```python
from build123d import *

# Parameters (mm, degrees)
CHAMFER1_SIZE       = 1
CHAMFER2_SIZE       = 0.5
SKETCH2_OUTSIDE_W   = 43.394
SKETCH2_OUTSIDE_H   = 43.394
SKETCH2_OUTSIDE_W_2 = 33.661520222
SKETCH2_OUTSIDE_H_2 = 15
CUT_EXTRUDE1_DEPTH  = 6


with BuildPart() as part:
    # Sketch1 → Revolve1 (revolve)
    with BuildSketch(Plane.XY):
        Polygon((3.5, -5), (3.5, 56), (6.5, 56), (6.5, 46), (10, 46), (10, 4), (13.5, 4), (13.5, 0), (6.25, 0), (6.25, -5), align=None)
    revolve(axis=Axis((0, 0, 0), (0, 1, 0)))

    # Chamfer1
    chamfer1_edges = [part.edges().sort_by_distance(p)[0] for p in [
        (-6.5, 56, 0),
    ]]
    chamfer(chamfer1_edges, length=CHAMFER1_SIZE)

    # Chamfer2
    chamfer2_edges = [part.edges().sort_by_distance(p)[0] for p in [
        (-10, 46, 0),
        (-3.5, 56, 0),
        (-3.5, -5, 0),
        (-6.25, -5, 0),
        (-13.5, 0, 0),
        (-13.5, 4, 0),
    ]]
    chamfer(chamfer2_edges, length=CHAMFER2_SIZE)

    # Sketch2 outside → Cut-Extrude1 (cut)
    with BuildSketch(Plane(origin=(0, 4, 0), x_dir=(1, 0, 0), z_dir=(0, 1, 0))):
        Rectangle(SKETCH2_OUTSIDE_W, SKETCH2_OUTSIDE_H)
        Rectangle(SKETCH2_OUTSIDE_W_2, SKETCH2_OUTSIDE_H_2, mode=Mode.SUBTRACT)
    extrude(amount=CUT_EXTRUDE1_DEPTH, mode=Mode.SUBTRACT)


solid = part.part
```
Check sheet for the modelled part. Datum: model origin and axes. Units: mm. A direction names the side the tool comes from. Give positions to 0.01 mm unless a question says otherwise; leave off trailing zeros. Write each loop counter-clockwise with the first axis right and the second up, starting at its lowest first coordinate (ties: lowest second). Pieces come first, ordered by that corner, then holes. Notation, with made-up numbers: (13, 70) - (30, 70) arc R6 ccw to (30, 81) - close; hole circle Ø3 at (-35.75, 62.5). An arc over 180 degrees is marked (long way). Answer as a JSON object with one key per item and string values. Group by question number.
1) Depth check by flat-ended pin: P1, Ø2, axis at x = -2, y = 40.5, coming from the -Z side; P2, Ø4, axis at y = 46, z = 3.5, coming from the -X side; P3, Ø6, axis at x = 9, z = -7.5, coming from the -Y side. Enter the tip coordinate at first touch or a pass-through.
2) Thickness scan on probe 1 along X at (y, z) = (33, 0); probe 2 along Y at (x, z) = (2.75, -10.5). Record the ranges inside material, lowest first. Write a range as from..to.
3) Sectioned sample at C-C (y = 35). Record the cut outline in (x, z), then the cut area to 3 significant figures.
4) Sectioned sample at B-B (y = 8). Record the cut outline in (x, z).
5) Access from +Z, -Z, +X, -X, +Y, -Y to the whole of each face (thin tool, end or side, straight path). Record for faces 1 (the face through (-4, 46, 6)), 2 (the face through (5.96, -2.28, -1.88)), 3 (the face through (0, 10, -8)), 4 (the face through (0, 4, 8)), 5 (the face through (0, 10, 8)).
6) Release check for a two-part mould opening along Z. For faces 6 (the face through (0, 7, 7.5)), 7 (the face through (-5.158, 50.437, 3.955)), 8 (the face through (0, 7, -7.5)), 9 (the face through (3.233, 25.92, 1.341)) record: pulls with the +Z half, pulls with the -Z half, needs draft (parallel to the pull), parting line crosses it, or undercut.
Geometry results:
{
 "1": {"P1": "stops at z = -9.95", "P2": "stops at x = -9.88", "P3": "stops at y = 0"},
 "2": {"probe 1": "x = -10..-3.5, 3.5..10", "probe 2": "y = 0..4"},
 "3": {"outline": "circle Ø20 at (0, 0); hole circle Ø7 at (0, 0)", "area": "276 mm^2"},
 "4": {"outline": "(-6.61, -7.5) - (6.61, -7.5) arc R10 ccw to (6.61, 7.5) - (-6.61, 7.5) arc R10 ccw to start; hole circle Ø7 at (0, 0)"},
 "5": {"face 1": "+Y", "face 2": "-Y", "face 3": "-Z, +X, -X", "face 4": "none", "face 5": "+Z, +X, -X"},
 "6": {"face 6": "pulls with the +Z half", "face 7": "parting line crosses it", "face 8": "pulls with the -Z half", "face 9": "undercut"}
}
